Autodesk Inventor part; units mm, degrees
ref_plane "YZ Plane" through (0, 0, 0) normal (1, 0, 0) x (0, 1, 0)
ref_plane "XZ Plane" through (0, 0, 0) normal (0, 1, 0) x (-1, 0, 0)
ref_plane "XY Plane" through (0, 0, 0) normal (0, 0, 1) x (1, 0, 0)
sketch "Sketch1 outline for Plate1" plane through (0, 0, 0) normal (0, 0, 1) x (1, 0, 0)
  line L0 (0, 25.4) -> (0, 0)
  line L1 (63.5, 25.4) -> (0, 25.4)
  line L2 (0, 0) -> (63.5, 0)
  line L3 (63.5, 0) -> (63.5, 25.4)
  circle A0 centre (28.575, 12.7) radius 2.4892
  circle A1 centre (53.975, 12.7) radius 2.4892
extrude "Plate1" add sketch "Sketch1 outline for Plate1" along normal blind 3.175
sketch "Sketch2" plane through (63.5, 26.67, -1.27) normal (0, 1, 0) x (-1, 0, 0)
  line L0 (63.5, 0) -> (0, 0)
  line L1 (0, 0) -> (0, -20.955)
  line L2 (0, -20.955) -> (63.5, -20.955)
  line L3 (63.5, -20.955) -> (63.5, 0)
edge flange "Flange1" height 25.4 angle 90 thickness 3.175 bend radius 1.27 thickness toward (0, 1, 0) relief tear relief width 3.175 relief depth 1.5875 corner gap 3.175 corner form 0 edges at (31.75, 25.4, 0) (31.75, 0, 0) wall of the first edge with corners at (0, 26.67, -1.27) (63.5, 26.67, -1.27) (63.5, 26.67, -22.225) (0, 26.67, -22.225)
bend "Bend1"
corner "Corner1"
sketch "Sketch1" plane through (0, 0, 0) normal (0, 0, 1) x (1, 0, 0)
  line L0 (0, 0) -> (75.688628, 0)
  line L1 (75.688628, -63.5) -> (0, -63.5)
  line L2 (20.955, 0) -> (25.144314, 0)
  line L3 (25.144314, 0) -> (25.144314, -3.175)
  line L4 (25.144314, -3.175) -> (20.955, -3.175)
  line L5 (20.955, -3.175) -> (20.955, 0)
  line L6 (20.955, -63.5) -> (20.955, 0)
  line L7 (25.144314, -63.5) -> (25.144314, 0)
  line L8 (20.955, -63.5) -> (25.144314, -63.5)
  line L9 (25.144314, -63.5) -> (25.144314, -60.325)
  line L10 (25.144314, -60.325) -> (20.955, -60.325)
  line L11 (20.955, -60.325) -> (20.955, -63.5)
  line L12 (50.544314, -63.5) -> (54.733628, -63.5)
  line L13 (54.733628, -63.5) -> (54.733628, -60.325)
  line L14 (54.733628, -60.325) -> (50.544314, -60.325)
  line L15 (50.544314, -60.325) -> (50.544314, -63.5)
  line L16 (50.544314, 0) -> (50.544314, -63.5)
  line L17 (54.733628, 0) -> (54.733628, -63.5)
  line L18 (50.544314, 0) -> (54.733628, 0)
  line L19 (54.733628, 0) -> (54.733628, -3.175)
  line L20 (54.733628, -3.175) -> (50.544314, -3.175)
  line L21 (50.544314, -3.175) -> (50.544314, 0)
  dimension "d10" = 12.7
  dimension "d11" = 28.575
sketch "Sketch3" plane through (0, -4.445, -22.225) normal (0, -1, 0) x (1, 0, 0)
  line L0 (0, 0) -> (0, 20.955)
  line L1 (63.5, 0) -> (0, 0)
  circle A0 centre (6.35, 9.525) radius 2.0701
  circle A1 centre (19.05, 9.525) radius 2.0701
  circle A2 centre (31.75, 9.525) radius 2.0701
  circle A3 centre (44.45, 9.525) radius 2.0701
  circle A4 centre (57.15, 9.525) radius 2.0701
  point P0 (0, 22.225)
  dimension "d23" = 4.1402
  dimension "d24" = 12.7
  dimension "d25" = 6.35
  dimension "d28" = 12.7
extrude "Extrusion1" cut sketch "Sketch3" against normal blind 50.8
equation "\"d13\" = BendReliefWidth"
equation "\"d14\" = BendReliefDepth"
equation "\"d15\" = MinimumRemnant"
equation "\"d16\" = BendRadius"
equation "\"d20\" = CornerReliefSize"
equation "\"d21\" = GapSize"
equation "\"d22\" = JacobiRadiusSize"
equation "\"BendRadius\" = Thickness"
equation "\"BendReliefWidth\" = Thickness"
equation "\"BendReliefDepth\" = 0.5 * Thickness"
equation "\"CornerReliefSize\" = 4 * Thickness"
equation "\"MinimumRemnant\" = 2 * Thickness"
equation "\"TransitionRadius\" = BendRadius"
equation "\"JacobiRadiusSize\" = BendRadius"
equation "\"GapSize\" = Thickness"
equation "\"d12\" = BendRadius"
properties part number "Side Mount Custom" material "Aluminum 6061"
Here's how the part is built. I have some questions about the finished solid (model axes, mm). A direction names the side the tool comes from. Round coordinates to 2 decimals unless told otherwise and drop trailing zeros. Loops run counter-clockwise (first coordinate to the right, second up) from the corner with the lowest first, then second, coordinate; pieces in that order, holes last.
1. Suppose I cut it at B-B, the plane z = -3. Please give me the cut outline in (x, y) (3 decimals).
Answers:
outline: (0, -4.445) - (63.5, -4.445) - (63.5, -1.27) - (0, -1.27) - close; (0, 26.67) - (63.5, 26.67) - (63.5, 29.845) - (0, 29.845) - close
2. Suppose I cut it at A-A, the plane x = 44.45. Please give me the cut outline in (y, z) (3 decimals).
Answers:
outline: (-4.445, -22.225) - (-1.27, -22.225) - (-1.27, -14.77) - (-4.445, -14.77) - close; (-4.445, -10.63) - (-1.27, -10.63) - (-1.27, -1.27) arc R1.27 cw to (0, 0) - (25.4, 0) arc R1.27 cw to (26.67, -1.27) - (26.67, -10.63) - (29.845, -10.63) - (29.845, -1.27) arc R4.445 ccw to (25.4, 3.175) - (0, 3.175) arc R4.445 ccw to (-4.445, -1.27) - close; (26.67, -22.225) - (29.845, -22.225) - (29.845, -14.77) - (26.67, -14.77) - close
3. Suppose I cut it at C-C, the plane z = -12.7. Give the number of separate pieces and of enclosed holes in the cut face, and give its area (3 significant figures).
Answers:
separate pieces: 12
enclosed holes: 0
area: 272 mm2
4. Suppose I cut it at D-D, the plane y = 16.5. Please give me the cut outline in (x, z) (3 decimals), and give its area (3 significant figures).
Answers:
outline: (0, 0) - (63.5, 0) - (63.5, 3.175) - (0, 3.175) - close
area: 202 mm2
5. Will these pins go through, and if not, where does the flat tip stop? pin 1 (3.5 mm diameter, centred on x = 44.45, z = -12.7, fed in from -Y); pin 2 (12.5 mm diameter, centred on x = 36, y = 12, fed in from -Z).
Answers:
pin 1: passes through
pin 2: stops at z = 0
6. Thinking about a two-plate mould opening in Z: for faces 3 (the face through (31.3, 12.9, 3.175)), 4 (the face through (30.95, 11.95, 1.57)), 5 (the face through (6.081, 28.235, -10.648)), which applies, released by +Z, released by -Z, zero draft, split by the parting line, or undercut?
Answers:
face 3: released by +Z
face 4: zero draft
face 5: undercut
7. If I drill on probe 1 along Y at (x, z) = (17, -17.5) (3 decimals); probe 2 along Z at (x, y) = (51, 16) (3 decimals); probe 3 along Y at (x, z) = (53.5, 2), over which ranges is the centre line in solid material (lowest first)?
Answers:
probe 1: y = -4.445 to -1.27, 26.67 to 29.845
probe 2: z = 0 to 3.175
probe 3: y = -3.01 to 10.26, 15.14 to 28.41
8. For faces 1 (the face through (29.68, -2.88, -12.61)), 2 (the face through (31.306, -0.908, -0.382)), which set-ups out of +Z, -Z, +X, -X, +Y, -Y let a thin tool reach every point of the face, with its end or its side?
Answers:
face 1: +Y, -Y
face 2: -Z, +X, -X
